For this review, take the finished solid that the model builds, in its own axes (mm). A direction names the side the tool comes from. Give positions to 0.01 mm unless a question says otherwise; leave off trailing zeros. Write each loop counter-clockwise with the first axis right and the second up, starting at its lowest first coordinate (ties: lowest second). Pieces come first, ordered by that corner, then holes. Notation, with made-up numbers: (78, 37) -> (84, 37) arc R25 ccw to (84, 73) -> close; hole circle Ø2 at (33.5, -20.5). An arc over 180 degrees is marked (long way). Return JSON: item names as keys, results as strings.
from build123d import *

# Parameters (mm, degrees)
SKETCH1_W           = 4
SKETCH1_H           = 40
EXTRUDE_THIN2_DEPTH = 18
SKETCH4_R           = 4
SKETCH7_R           = 2.2
CUT_EXTRUDE2_DEPTH  = 45.586993619
SKETCH8_R           = 4.03
CUT_EXTRUDE5_DEPTH  = 20
SKETCH9_R           = 1.5
CUT_EXTRUDE6_DEPTH  = 45.045431091
FILLET1_R           = 10


with BuildPart() as part:
    # Sketch1 → Extrude-Thin2 (new body)
    with BuildSketch(Plane.XY):
        with Locations((2, 20)):
            Rectangle(SKETCH1_W, SKETCH1_H)
    extrude(amount=EXTRUDE_THIN2_DEPTH)

    # Sweep3: sweep along a curve in space
    with BuildLine() as sweep3_path:
        Line((4, 0, 0), (4, 40, 0))
    # Sketch4 → Sweep3 (sweep)
    with BuildSketch(Plane(origin=(0, 40, 0), x_dir=(1, 0, 0), z_dir=(0, 1, 0))):
        with Locations((4, 0)):
            Circle(SKETCH4_R)
    sweep(path=sweep3_path.line)

    # Sketch7 → Cut-Extrude2 (cut, through all)
    with BuildSketch(Plane(origin=(0, 40, 0), x_dir=(1, 0, 0), z_dir=(0, 1, 0))):
        with Locations(Location((4, 0, 0), (0, 0, 270))):
            Circle(SKETCH7_R)
    extrude(amount=-CUT_EXTRUDE2_DEPTH, mode=Mode.SUBTRACT)

    # Sketch8 → Cut-Extrude5 (cut)
    with BuildSketch(Plane(origin=(0, 40, 0), x_dir=(1, 0, 0), z_dir=(0, 1, 0))):
        with Locations((4, 0)):
            Circle(SKETCH8_R)
    extrude(amount=-CUT_EXTRUDE5_DEPTH, mode=Mode.SUBTRACT)

    # Sketch9 → Cut-Extrude6 (cut, through all)
    with BuildSketch(Plane(origin=(4, 0, 0), x_dir=(0, 0, -1), z_dir=(1, 0, 0))):
        with Locations((-11.5, 10)):
            Circle(SKETCH9_R)
        with Locations((-11.5, 30)):
            Circle(SKETCH9_R)
    extrude(amount=-CUT_EXTRUDE6_DEPTH, mode=Mode.SUBTRACT)

    # Fillet1
    fillet1_edges = [part.edges().sort_by_distance(p)[0] for p in [
        (2, 0, 18),
        (2, 40, 18),
    ]]
    fillet(fillet1_edges, radius=FILLET1_R)


solid = part.part
1. Add section C-C, the plane z = -1. State the section outline as (x, y) points, plus the area to 3 significant figures.
Results found:
{"outline": "(0.13, 0) -> (2.04, 0) -> (2.04, 20) -> (0.13, 20) -> close; (5.96, 0) -> (7.87, 0) -> (7.87, 20) -> (5.96, 20) -> close", "area": "76.5 mm²"}
2. Add section B-B, the plane y = 4. State the section outline as (x, z) points, plus the area to 3 significant figures.
Results found:
{"outline": "(0, 0) arc R4 ccw (long way) to (4, 4) -> (4, 16) -> (0, 16) -> close; hole circle Ø4.4 at (4, 0)", "area": "86.5 mm²"}
3. The part is to be moulded in two halves that separate along Y. For faces 4 (the flat face through (2, 0, 2)), 5 (the cylindrical face through (2, 9.1, 12.7)), 6 (the flat face through (6, 20, 2)), say which applies: +Y half, -Y half, draft (parallel to the pull), parting line (faces both ways), or undercut.
Results found:
{"face 4": "-Y half", "face 5": "undercut", "face 6": "+Y half"}
4. For faces 1 (the cylindrical face through (6.92, 10.14, -2.734)), 2 (the flat face through (4, 20, 11)), 3 (the cylindrical face through (1.3, 30.14, 2.99)), list the 3-axis set-ups (+Z, -Z, +X, -X, +Y, -Y) from which the entire face can be reached by the end or side of a thin tool; tool diameter is ignored.
Results found:
{"face 1": "+Y, -Y", "face 2": "+Z, +X, +Y, -Y", "face 3": "-Z, +X, +Y"}
5. Add section A-A, the plane x = 2.5. State the section outline as (y, z) points, plus the area to 3 significant figures.
Results found:
{"outline": "(0, -3.71) -> (20, -3.71) -> (20, -1.61) -> (0, -1.61) -> close; (0, 1.61) -> (20, 1.61) -> (20, 3.74) -> (40, 3.74) -> (40, 8) arc R10 ccw to (30, 18) -> (10, 18) arc R10 ccw to (0, 8) -> close; hole circle Ø3 at (10, 11.5); hole circle Ø3 at (30, 11.5)", "area": "598 mm²"}
6. Add section D-D, the plane y = 9.5. State the section outline as (x, z) points.
Results found:
{"outline": "(0, 0) arc R4 ccw (long way) to (4, 4) -> (4, 10.09) -> (0, 10.09) -> close; (0, 12.91) -> (4, 12.91) -> (4, 17.99) -> (0, 17.99) -> close; hole circle Ø4.4 at (4, 0)"}
7. To check wall thickness, follow probe 1 along Y at (x, z) = (0.9, 11.5); probe 2 along X at (y, z) = (35, 10); probe 3 along Z at (x, y) = (2.5, 19). State the ranges of each line that lie inside material, in increasing order.
Results found:
{"probe 1": "y = 0.63 to 8.5, 11.5 to 28.5, 31.5 to 39.37", "probe 2": "x = 0 to 4", "probe 3": "z = -3.71 to -1.61, 1.61 to 18"}
8. For pin 1 (3 mm diameter, centred on y = 24.5, z = -2, fed in from -X); pin 2 (4 mm diameter, centred on x = 3, y = 32.5, fed in from -Z); pin 3 (7 mm diameter, centred on y = 16.5, z = 14.5, fed in from +X); pin 4 (3 mm diameter, centred on x = 5.5, z = 0, fed in from +Y), all flat-tipped, find the tip position at first contact; note any pin that passes through.
Results found:
{"pin 1": "passes through", "pin 2": "stops at z = 2.69", "pin 3": "stops at x = 4", "pin 4": "stops at y = 20"}
